Here's how the part is built. I have some questions about the finished solid (model axes, mm). A direction names the side the tool comes from. Coordinates: 2 decimals unless noted, no trailing zeros. Loops run counter-clockwise (first coordinate to the right, second up) from the corner with the lowest first, then second, coordinate; pieces in that order, holes last. Notation, with made-up numbers: (-7.5, 3.5) -> (29.5, 3.5) arc R25 ccw to (29.5, 24.5) -> close; hole circle Ø1 at (-4.5, 28). An arc over 180 degrees is marked (long way). Answer as a JSON object with one key per item and string values. Group by question number.
1) I'm going to push flat-ended pins straight in: pin 1 (8 mm diameter, centred on y = -3.5, z = 3, fed in from +X); pin 2 (4 mm diameter, centred on y = -5.5, z = -1, fed in from -X); pin 3 (0.9 mm diameter, centred on y = 4.5, z = 3.5, fed in from +X); pin 4 (8 mm diameter, centred on y = -8, z = 7.5, fed in from -X). Where does each tip first touch, or does it pass through?
2) I need wall thicknesses on probe 1 along Z at (x, y) = (7, 4.75); probe 2 along X at (y, z) = (8.75, 0.5). Which ranges of each line are inside material? Lowest first, please. Write a range as [from, to].
3) If we mould it in two halves opening along X, with no side actions, what happens to faces 1 (the flat face through (6, 6, 0)), 2 (the flat face through (0, 0, 0)), 3 (the flat face through (10.2, 0.1, 4))? For each: +X half, -X half, draft (parallel to the pull), parting line (faces both ways), or undercut.
4) I want a section at A-A (y = -3). Write out the boundary of the cut face in (x, z).
5) Which directions (+Z, -Z, +X, -X, +Y, -Y) give clear straight access to the entire face, cutting with the end or side of a thin tool? Please do faces 4 (the flat face through (4, 4, 0)), 5 (the flat face through (2, 4, 0)), 6 (the flat face through (7, 0, 2.5)), 7 (the flat face through (7, 0, -2.5)), 8 (the flat face through (5, -2.5, 0)).
6) I want a section at C-C (y = -0.25). Write out the boundary of the cut face in (x, z), then the cut area to 3 significant figures.
7) I want a section at D-D (z = -3.5). Write out the boundary of the cut face in (x, y).
8) I want a section at B-B (z = -1). Write out the boundary of the cut face in (x, y).
```python
from build123d import *

# Parameters (mm, degrees)
BOSS_EXTRU_1_DEPTH = 10
BOSS_EXTRU_2_DEPTH = 10


with BuildPart() as part:
    # ProfileRainureEsquisse → Boss.-Extru.1 (new body, symmetric)
    with BuildSketch(Plane.XY):
        Polygon((0, -2.5), (0, 2.5), (4, 5.5), (4, 2.5), (6, 2.5), (6, -2.5), (4, -2.5), (4, -5.5), align=None)
    extrude(amount=BOSS_EXTRU_1_DEPTH, both=True)

    # Esquisse1 → Boss.-Extru.2 (add, symmetric)
    with BuildSketch(Plane(origin=(0, 0, 0), x_dir=(1, 0, 0), z_dir=(0, 1, 0))):
        Polygon((6, 2.5), (8.2, 2.5), (8.2, 5.5), (12.2, 2.5), (12.2, -2.5), (8.2, -5.5), (8.2, -2.5), (6, -2.5), align=None)
    extrude(amount=BOSS_EXTRU_2_DEPTH, both=True)


solid = part.part
```
Determined:
{
 "1": {"pin 1": "x = 12.2", "pin 2": "x = 1.33", "pin 3": "x = 11.47", "pin 4": "x = 2"},
 "2": {"probe 1": "[-2.5, 2.5]", "probe 2": "[6, 12.2]"},
 "3": {"face 1": "undercut", "face 2": "-X half", "face 3": "+X half"},
 "4": {"outline": "(0.67, -10) -> (4, -10) -> (4, 10) -> (0.67, 10) -> close; (6, -2.5) -> (8.2, -2.5) -> (8.2, -5.5) -> (12.2, -2.5) -> (12.2, 2.5) -> (8.2, 5.5) -> (8.2, 2.5) -> (6, 2.5) -> close"},
 "5": {"face 4": "+Z, -Z, +Y", "face 5": "+Z, -Z, -X, +Y", "face 6": "+Z, +Y, -Y", "face 7": "-Z, +Y, -Y", "face 8": "+Z, -Z, -Y"},
 "6": {"outline": "(0, -10) -> (6, -10) -> (6, -2.5) -> (8.2, -2.5) -> (8.2, -5.5) -> (12.2, -2.5) -> (12.2, 2.5) -> (8.2, 5.5) -> (8.2, 2.5) -> (6, 2.5) -> (6, 10) -> (0, 10) -> close", "area": "163 mm^2"},
 "7": {"outline": "(0, -2.5) -> (4, -5.5) -> (4, -2.5) -> (6, -2.5) -> (6, 2.5) -> (4, 2.5) -> (4, 5.5) -> (0, 2.5) -> close; (8.2, -10) -> (10.87, -10) -> (10.87, 10) -> (8.2, 10) -> close"},
 "8": {"outline": "(0, -2.5) -> (4, -5.5) -> (4, -2.5) -> (6, -2.5) -> (6, -10) -> (12.2, -10) -> (12.2, 10) -> (6, 10) -> (6, 2.5) -> (4, 2.5) -> (4, 5.5) -> (0, 2.5) -> close"}
}
